Read the model definition and answer for the solid it produces. Units are mm, in the model's axes. Face numbers are marked on the shaded views. Coordinates: 2 decimals unless noted, no trailing zeros. Order: outer loops, then holes, each group sorted by start corner. A loop starts at its lowest first (then second) coordinate and runs counter-clockwise, first axis right, second up. Notation, with made-up numbers: M -4.75,36 L 21.25,36 A25 cw 21.25,70 Z; hole C 21,65.25 d3. An arc over 180 degrees is marked long. One line per question, with ' | ' between items. Start each with the question number.
1) Consider probe 1 along X at (y, z) = (0.2, 3.5). Determine where the line is inside the solid, lowest interval first.
2) Find section D-D, the plane x = 7.5. Write down the section's boundary in (y, z) (3 decimals), plus the area to 4 significant figures.
3) Find section B-B, the plane z = 0. Write down the section's boundary in (x, y) (3 decimals).
4) Find section C-C, the plane x = 2.75. Write down the section's boundary in (y, z) (3 decimals).
5) Find section A-A, the plane x = 0. Write down the section's boundary in (y, z) (3 decimals).
6) Given P1, Ø5, axis at x = -3, z = -5, coming from the +Y side (3 decimals); P2, Ø7.5, axis at x = -2.5, z = 3, coming from the +Y side, each flat-ended and moving along its own axis, determine where each tip first touches the part or whether it passes through.
7) The mould has two halves that part along Z. Classify the marked faces 1, 2 and 3: +Z half, -Z half, draft (parallel to the pull), parting line (faces both ways), or undercut.
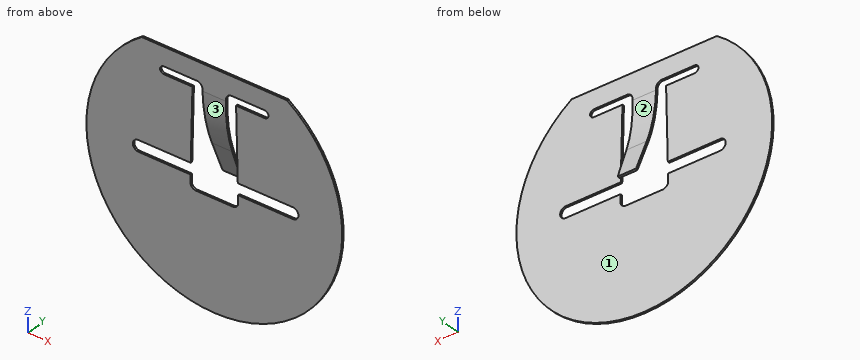
from build123d import *

# Parameters (mm, degrees)
EXTRUDE1_DEPTH = 0.125
SKETCH3_W      = 1.6
SKETCH3_H      = 0.125
EXTRUDE2_DEPTH = 2.616620884
FILLET3_R      = 0.365


with BuildPart() as part:
    # Sketch1 → Extrude1 (new body)
    with BuildSketch(Plane(origin=(0, 0, 0), x_dir=(1, 0, 0), z_dir=(0, 1, 0))):
        with BuildLine():
            Line((4.82182538, -7), (-4.82182538, -7))
            ThreePointArc((-4.82182538, -7), (0, 8.5), (4.82182538, -7))
        make_face()
        with BuildLine():
            Line((1.5625, -0.375), (5.215, -0.375))
            ThreePointArc((5.215, -0.375), (5.59, 0), (5.215, 0.375))
            Line((5.215, 0.375), (1.579807692, 0.375))
            Line((1.579807692, 0.375), (1.591146503, 0.866348457))
            ThreePointArc((1.591146503, 0.866348457), (1.484452699, 1.137088412), (1.216246315, 1.25))
            Line((1.216246315, 1.25), (-1.216246315, 1.25))
            ThreePointArc((-1.216246315, 1.25), (-1.484452699, 1.137088412), (-1.591146503, 0.866348457))
            Line((-1.591146503, 0.866348457), (-1.579807692, 0.375))
            Line((-1.579807692, 0.375), (-5.035, 0.375))
            ThreePointArc((-5.035, 0.375), (-5.41, 0), (-5.035, -0.375))
            Line((-5.035, -0.375), (-1.5625, -0.375))
            Line((-1.5625, -0.375), (-1.45, -5.25))
            Line((-1.45, -5.25), (-3.35, -5.25))
            ThreePointArc((-3.35, -5.25), (-3.6, -5.5), (-3.35, -5.75))
            Line((-3.35, -5.75), (3.35, -5.75))
            ThreePointArc((3.35, -5.75), (3.6, -5.5), (3.35, -5.25))
            Line((3.35, -5.25), (1.45, -5.25))
            Line((1.45, -5.25), (1.5625, -0.375))
        make_face(mode=Mode.SUBTRACT)
    extrude(amount=EXTRUDE1_DEPTH)

    # Sweep2: sweep along a path in Sketch2
    with BuildLine(Plane(origin=(0, 0, 0), x_dir=(0, 0, -1), z_dir=(1, 0, 0))) as sweep2_path:
        Line((0.5, 1.5), (-1.650382858, 0.670329243))
        ThreePointArc((-1.650382858, 0.670329243), (-3.419249821, 0.169010539), (-5.25, 0))
        Line((-5.25, 0), (-5.75, 0))
    # Sketch3 → Sweep2 (sweep)
    with BuildSketch(Plane(origin=(0, 0, 5.75), x_dir=(-1, 0, 0), z_dir=(0, 0, -1))):
        with Locations((0, 0.0625)):
            Rectangle(SKETCH3_W, SKETCH3_H)
    sweep(path=sweep2_path.line)

    # Sketch5 → Extrude2 (cut, through all)
    with BuildSketch(Plane(origin=(0, 0, 0), x_dir=(1, 0, 0), z_dir=(0, 1, 0))):
        Polygon((-0.6, 0.75), (-0.8, -5.75), (-1.2, -5.75), (-1.2, 1), (1.2, 1), (1.2, -5.75), (0.8, -5.75), (0.6, 0.75), align=None)
    extrude(amount=EXTRUDE2_DEPTH, mode=Mode.SUBTRACT)

    # Fillet3
    fillet3_edges = [part.edges().sort_by_distance(p)[0] for p in [
        (0.8, 0.0625, 5.75),
        (-0.8, 0.0625, 5.75),
    ]]
    fillet(fillet3_edges, radius=FILLET3_R)


solid = part.part
Report:
1) probe 1: x = -0.73 to 0.73
2) outline: M 0,-4 L 0.125,-4 L 0.125,4 L 0,4 Z | area: 1.000 mm^2
3) outline: M -8.5,0 L -5.41,0 L -5.41,0.125 L -8.5,0.125 Z; M -0.623,1.307 L 0.623,1.307 L 0.623,1.441 L -0.623,1.441 Z; M 5.59,0 L 8.5,0 L 8.5,0.125 L 5.59,0.125 Z
4) outline: M 0,-8.043 L 0.125,-8.043 L 0.125,-0.375 L 0,-0.375 Z; M 0,0.375 L 0.125,0.375 L 0.125,5.25 L 0,5.25 Z; M 0,5.75 L 0.125,5.75 L 0.125,7 L 0,7 Z
5) outline: M 0,-8.5 L 0.125,-8.5 L 0.125,-1.25 L 0,-1.25 Z; M 0,5.25 A10 ccw 0.67,1.65 L 1.5,-0.5 L 1.617,-0.455 L 0.787,1.695 A9.875 cw 0.125,5.25 L 0.125,7 L 0,7 Z
6) P1: stops at y = 0.125 | P2: stops at y = 1.53
7) face 1: draft | face 2: +Z half | face 3: undercut
